from build123d import *

# Parameters (mm, degrees)
BOSS_EXTRUDE1_DEPTH = 6.35
SKETCH2_R           = 2.25
SKETCH2_R_2         = 30
CUT_EXTRUDE1_DEPTH  = 7.35
SKETCH6_R           = 0.85
CUT_EXTRUDE5_DEPTH  = 7.35
SKETCH8_R           = 25
CUT_EXTRUDE9_DEPTH  = 7.35
SKETCH9_R           = 1.65
CUT_EXTRUDE10_DEPTH = 30
CUT_EXTRUDE12_DEPTH = 30
SKETCH10_R          = 1.65
CUT_EXTRUDE13_DEPTH = 10


with BuildPart() as part:
    # Sketch1 → Boss-Extrude1 (new body)
    with BuildSketch(Plane(origin=(0, 0, 0), x_dir=(1, 0, 0), z_dir=(0, 1, 0))):
        Polygon((-71, 140), (71, 140), (71, -140), (-131, -140), (-131, 120), (-71, 120), align=None)
    extrude(amount=BOSS_EXTRUDE1_DEPTH)

    # Sketch2 → Cut-Extrude1 (cut, through all)
    with BuildSketch(Plane(origin=(0, 6.35, 0), x_dir=(1, 0, 0), z_dir=(0, 1, 0))):
        with Locations((0, -23.5)):
            Circle(SKETCH2_R)
        with Locations((29.344931419, -35.655068581)):
            Circle(SKETCH2_R)
        with Locations((41.5, -65)):
            Circle(SKETCH2_R)
        with Locations((29.344931419, -94.344931419)):
            Circle(SKETCH2_R)
        with Locations((0, -106.5)):
            Circle(SKETCH2_R)
        with Locations((-29.344931419, -94.344931419)):
            Circle(SKETCH2_R)
        with Locations((-41.5, -65)):
            Circle(SKETCH2_R)
        with Locations((-29.344931419, -35.655068581)):
            Circle(SKETCH2_R)
        with Locations((0, -65)):
            Circle(SKETCH2_R_2)
    extrude(amount=-CUT_EXTRUDE1_DEPTH, mode=Mode.SUBTRACT)

    # Sketch6 → Cut-Extrude5 (cut, through all)
    with BuildSketch(Plane(origin=(0, 6.35, 0), x_dir=(1, 0, 0), z_dir=(0, 1, 0))):
        with Locations((-36.963798099, -42.522452757)):
            Circle(SKETCH6_R)
        with Locations((-40.978671586, -51.132376734)):
            Circle(SKETCH6_R)
        with Locations((-29.908156972, -51.053597363)):
            Circle(SKETCH6_R)
    extrude(amount=-CUT_EXTRUDE5_DEPTH, mode=Mode.SUBTRACT)

    # Sketch8 → Cut-Extrude9 (cut, through all)
    with BuildSketch(Plane(origin=(0, 6.35, 0), x_dir=(1, 0, 0), z_dir=(0, 1, 0))):
        with Locations((0, 65)):
            Circle(SKETCH8_R)
    extrude(amount=-CUT_EXTRUDE9_DEPTH, mode=Mode.SUBTRACT)

    # Sketch9 → Cut-Extrude10 (cut)
    with BuildSketch(Plane(origin=(0, 0, 0), x_dir=(-1, 0, 0), z_dir=(0, -1, 0))):
        with Locations((45.6, 129.325)):
            Circle(SKETCH9_R)
        with Locations((5.6, 129.325)):
            Circle(SKETCH9_R)
        with Locations((-34.4, 129.325)):
            Circle(SKETCH9_R)
        with Locations((65.6, 129.325)):
            Circle(SKETCH9_R)
        with Locations((25.6, 129.325)):
            Circle(SKETCH9_R)
        with Locations((-14.4, 129.325)):
            Circle(SKETCH9_R)
        with Locations((-54.4, 129.325)):
            Circle(SKETCH9_R)
    extrude(amount=-CUT_EXTRUDE10_DEPTH, mode=Mode.SUBTRACT)

    # Sketch11 → Cut-Extrude12 (cut)
    with BuildSketch(Plane(origin=(0, 6.35, 0), x_dir=(1, 0, 0), z_dir=(0, 1, 0))):
        with BuildLine():
            Line((-63.95, -128.355), (-63.95, -131.655))
            ThreePointArc((-63.95, -131.655), (-65.6, -133.305), (-67.25, -131.655))
            Line((-67.25, -131.655), (-67.25, -128.355))
            ThreePointArc((-67.25, -128.355), (-65.6, -126.705), (-63.95, -128.355))
        make_face()
        with BuildLine():
            Line((-23.95, -128.353535871), (-23.95, -131.653535871))
            ThreePointArc((-23.95, -131.653535871), (-25.6, -133.303535871), (-27.25, -131.653535871))
            Line((-27.25, -131.653535871), (-27.25, -128.353535871))
            ThreePointArc((-27.25, -128.353535871), (-25.6, -126.703535871), (-23.95, -128.353535871))
        make_face()
        with BuildLine():
            Line((16.05, -128.352071742), (16.05, -131.652071742))
            ThreePointArc((16.05, -131.652071742), (14.4, -133.302071742), (12.75, -131.652071742))
            Line((12.75, -131.652071742), (12.75, -128.352071742))
            ThreePointArc((12.75, -128.352071742), (14.4, -126.702071742), (16.05, -128.352071742))
        make_face()
        with BuildLine():
            Line((56.05, -128.350607613), (56.05, -131.650607613))
            ThreePointArc((56.05, -131.650607613), (54.4, -133.300607613), (52.75, -131.650607613))
            Line((52.75, -131.650607613), (52.75, -128.350607613))
            ThreePointArc((52.75, -128.350607613), (54.4, -126.700607613), (56.05, -128.350607613))
        make_face()
    extrude(amount=-CUT_EXTRUDE12_DEPTH, mode=Mode.SUBTRACT)

    # Sketch10 → Cut-Extrude13 (cut)
    with BuildSketch(Plane.XZ):
        with Locations((-120.325, -110)):
            Circle(SKETCH10_R)
        with BuildLine():
            Line((-118.675, -108.35), (-120.325, -108.35))
            ThreePointArc((-120.325, -108.35), (-119.158273811, -108.833273811), (-118.675, -110))
            ThreePointArc((-118.675, -110), (-119.158273801, -111.166726179), (-120.324999972, -111.65))
            Line((-120.324999972, -111.65), (-118.675, -111.65))
            ThreePointArc((-118.675, -111.65), (-117.025, -110), (-118.675, -108.35))
        make_face()
        with BuildLine():
            Line((-120.325, -108.35), (-121.975, -108.35))
            ThreePointArc((-121.975, -108.35), (-123.625, -110), (-121.975, -111.65))
            Line((-121.975, -111.65), (-120.324999972, -111.65))
            ThreePointArc((-120.324999972, -111.65), (-121.975, -110.000000014), (-120.325, -108.35))
        make_face()
        with BuildLine():
            Line((-120.325, -48.35), (-121.975, -48.35))
            ThreePointArc((-121.975, -48.35), (-123.625, -50), (-121.975, -51.65))
            Line((-121.975, -51.65), (-120.325, -51.65))
            ThreePointArc((-120.325, -51.65), (-121.975, -50), (-120.325, -48.35))
        make_face()
        with Locations((-120.325, -50)):
            Circle(SKETCH10_R)
        with BuildLine():
            Line((-118.675, -48.35), (-120.325, -48.35))
            ThreePointArc((-120.325, -48.35), (-119.158273811, -48.833273811), (-118.675, -50))
            ThreePointArc((-118.675, -50), (-119.158273811, -51.166726189), (-120.325, -51.65))
            Line((-120.325, -51.65), (-118.675, -51.65))
            ThreePointArc((-118.675, -51.65), (-117.025, -50), (-118.675, -48.35))
        make_face()
        with BuildLine():
            Line((-120.325, 11.65), (-121.975, 11.65))
            ThreePointArc((-121.975, 11.65), (-123.625, 10), (-121.975, 8.35))
            Line((-121.975, 8.35), (-120.325, 8.35))
            ThreePointArc((-120.325, 8.35), (-121.975, 10), (-120.325, 11.65))
        make_face()
        with Locations((-120.325, 10)):
            Circle(SKETCH10_R)
        with BuildLine():
            Line((-118.675, 11.65), (-120.325, 11.65))
            ThreePointArc((-120.325, 11.65), (-119.158273811, 11.166726189), (-118.675, 10))
            ThreePointArc((-118.675, 10), (-119.158273811, 8.833273811), (-120.325, 8.35))
            Line((-120.325, 8.35), (-118.675, 8.35))
            ThreePointArc((-118.675, 8.35), (-117.025, 10), (-118.675, 11.65))
        make_face()
        with BuildLine():
            Line((-120.325, 71.65), (-121.975, 71.65))
            ThreePointArc((-121.975, 71.65), (-123.625, 70), (-121.975, 68.35))
            Line((-121.975, 68.35), (-120.325, 68.35))
            ThreePointArc((-120.325, 68.35), (-121.975, 70), (-120.325, 71.65))
        make_face()
        with Locations((-120.325, 70)):
            Circle(SKETCH10_R)
        with BuildLine():
            Line((-118.675, 71.65), (-120.325, 71.65))
            ThreePointArc((-120.325, 71.65), (-119.158273811, 71.166726189), (-118.675, 70))
            ThreePointArc((-118.675, 70), (-119.158273811, 68.833273811), (-120.325, 68.35))
            Line((-120.325, 68.35), (-118.675, 68.35))
            ThreePointArc((-118.675, 68.35), (-117.025, 70), (-118.675, 71.65))
        make_face()
    extrude(amount=-CUT_EXTRUDE13_DEPTH, mode=Mode.SUBTRACT)


solid = part.part
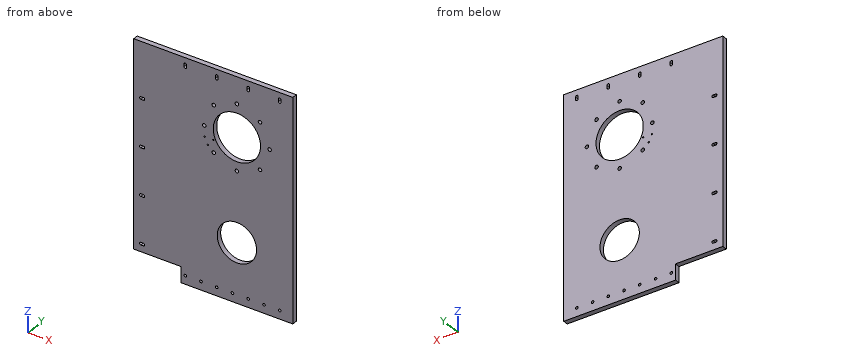
The listing builds one solid part. Answer for the finished solid, in the listing's coordinates (mm). Give positions to 0.01 mm unless a question says otherwise; leave off trailing zeros. Loops run counter-clockwise (first coordinate to the right, second up) from the corner with the lowest first, then second, coordinate; pieces in that order, holes last. Notation, with made-up numbers: (73.25, 40) - (82.25, 40) arc R35 ccw to (82.25, 74) - close; hole circle Ø9 at (-5.75, 34). An arc over 180 degrees is marked (long way). Write each question's results on one line, items separated by ' | '.
1. Consider probe 1 along X at (y, z) = (4.75, 106.5); probe 2 along Z at (x, y) = (14.4, 2.75) (3 decimals); probe 3 along Z at (x, y) = (-25.6, 2.25) (3 decimals). Determine where each line is inside the solid, lowest interval first. Write a range as from..to.
Resolved:
probe 1: x = -131..-2.25, 2.25..71 | probe 2: z = -140..-130.975, -127.675..-85.436, -44.564..38.682, 91.318..126.702, 133.302..140 | probe 3: z = -140..-130.975, -127.675..49.359, 80.641..126.704, 133.304..140
2. Flat-ended cylindrical pins translate along their axes: P1, Ø1.5, axis at x = -40.98, z = 51.13, coming from the -Y side; P2, Ø3.5, axis at x = -120.5, y = 2, coming from the -Z side. Find the tip coordinate at first contact, or state that the pin passes through.
Resolved:
P1: passes through | P2: stops at z = -120
3. Find section C-C, the plane x = -88. Write down the section's boundary in (y, z).
Resolved:
outline: (0, -120) - (6.35, -120) - (6.35, 140) - (0, 140) - close
4. Find section B-B, the plane x = -21. Write down the section's boundary in (y, z).
Resolved:
outline: (0, -140) - (6.35, -140) - (6.35, -78.56) - (0, -78.56) - close; (0, -51.44) - (6.35, -51.44) - (6.35, 43.58) - (0, 43.58) - close; (0, 86.42) - (6.35, 86.42) - (6.35, 140) - (0, 140) - close
5. Find section A-A, the plane z = 74.5. Write down the section's boundary in (x, y).
Resolved:
outline: (-131, 0) - (-28.46, 0) - (-28.46, 6.35) - (-131, 6.35) - close; (28.46, 0) - (71, 0) - (71, 6.35) - (28.46, 6.35) - close
6. Find section D-D, the plane y = 3.25. Count the separate pieces of the cut face and the enclosed holes in it, then the cut area to 3 significant figures.
Resolved:
separate pieces: 1 | enclosed holes: 28 | area: 50,200 mm^2
